from build123d import *

# Parameters (mm, degrees)
SKETCH1_W                        = 149.225
SKETCH1_H                        = 76.2
BASE_FLANGE1_DEPTH               = 3.175
EDGE_FLANGE1_STRIP_W             = 19.05
EDGE_FLANGE1_STRIP_H             = 3.175
EDGE_FLANGE1_STRIP_CUT_DEPTH     = 149.225
EDGE_FLANGE1_STRIP_2_W           = 19.05
EDGE_FLANGE1_STRIP_2_H           = 3.175
EDGE_FLANGE1_STRIP_CUT_2_DEPTH   = 149.225
EDGE_FLANGE1_DEPTH               = 149.225
EDGE_FLANGE1_BEND_DEPTH          = 149.225
SKETCH17_W                       = 25.4
SKETCH17_H                       = 9.525
CUT_EXTRUDE1_DEPTH               = 110.04244332
EDGE_FLANGE2_STRIP_W             = 19.05
EDGE_FLANGE2_STRIP_H             = 3.175
EDGE_FLANGE2_STRIP_CUT_DEPTH     = 123.825
EDGE_FLANGE2_STRIP_2_W           = 19.05
EDGE_FLANGE2_STRIP_2_H           = 3.175
EDGE_FLANGE2_STRIP_CUT_2_DEPTH   = 123.825
EDGE_FLANGE2_DEPTH               = 123.825
EDGE_FLANGE2_BEND_DEPTH          = 123.825
SKETCH18_R                       = 2.3876
CUT_EXTRUDE2_DEPTH               = 97.614069214
LPATTERN1_COUNT                  = 2
LPATTERN1_PITCH                  = 98.425
LPATTERN1_COUNT_DIR2             = 2
LPATTERN1_PITCH_DIR2             = 95.25
FILLET1_R                        = 3.175
F_10_0_1935_DIAMETER_HOLE1_D     = 4.9149
F_10_0_1935_DIAMETER_HOLE1_DEPTH = 3.175


# Sheet-metal steps are written as plain solids
with BuildPart() as part:
    # Sketch1 → Base-Flange1 (new body)
    with BuildSketch(Plane.XY):
        Rectangle(SKETCH1_W, SKETCH1_H)
    extrude(amount=-BASE_FLANGE1_DEPTH)

    # Edge-Flange1 strip (across the edge) → Edge-Flange1 strip cut (cut)
    with BuildSketch(Plane(origin=(74.6125, -38.1, -3.175), x_dir=(0, 1, 0), z_dir=(-1, 0, 0))):
        with Locations((-3.175, -1.5875)):
            Rectangle(EDGE_FLANGE1_STRIP_W, EDGE_FLANGE1_STRIP_H)
    extrude(amount=EDGE_FLANGE1_STRIP_CUT_DEPTH, mode=Mode.SUBTRACT)

    # Edge-Flange1 strip 2 (across the edge) → Edge-Flange1 strip cut 2 (cut)
    with BuildSketch(Plane(origin=(-74.6125, 38.1, -3.175), x_dir=(0, -1, 0), z_dir=(1, 0, 0))):
        with Locations((-3.175, -1.5875)):
            Rectangle(EDGE_FLANGE1_STRIP_2_W, EDGE_FLANGE1_STRIP_2_H)
    extrude(amount=EDGE_FLANGE1_STRIP_CUT_2_DEPTH, mode=Mode.SUBTRACT)

    # Edge-Flange1 section (across the edge) → Edge-Flange1 (add)
    with BuildSketch(Plane(origin=(74.6125, -38.1, -3.175), x_dir=(0, 1, 0), z_dir=(-1, 0, 0))):
        with BuildLine():
            Line((0, 3.175), (0, 19.558))
            Line((0, 19.558), (3.175, 19.558))
            Line((3.175, 19.558), (3.175, 3.175))
            ThreePointArc((3.175, 3.175), (4.10493597, 0.92993597), (6.35, 0))
            Line((6.35, 0), (6.35, -3.175))
            ThreePointArc((6.35, -3.175), (1.859871939, -1.315128061), (0, 3.175))
        make_face()
    extrude(amount=EDGE_FLANGE1_DEPTH)

    # Edge-Flange1 section 2 (across the edge) → Edge-Flange1 bend (add)
    with BuildSketch(Plane(origin=(-74.6125, 38.1, -3.175), x_dir=(0, -1, 0), z_dir=(1, 0, 0))):
        with BuildLine():
            Line((0, 3.175), (0, 19.558))
            Line((0, 19.558), (3.175, 19.558))
            Line((3.175, 19.558), (3.175, 3.175))
            ThreePointArc((3.175, 3.175), (4.10493597, 0.92993597), (6.35, 0))
            Line((6.35, 0), (6.35, -3.175))
            ThreePointArc((6.35, -3.175), (1.859871939, -1.315128061), (0, 3.175))
        make_face()
    extrude(amount=EDGE_FLANGE1_BEND_DEPTH)

    # Sketch17 → Cut-Extrude1 (cut, through all)
    with BuildSketch(Plane.XZ.offset(38.1)):
        with Locations((-61.9125, -17.9705)):
            Rectangle(SKETCH17_W, SKETCH17_H)
    extrude(amount=-CUT_EXTRUDE1_DEPTH, mode=Mode.SUBTRACT)

    # Edge-Flange2 strip (across the edge) → Edge-Flange2 strip cut (cut)
    with BuildSketch(Plane(origin=(-49.2125, -38.1, -22.733), x_dir=(0, 0, 1), z_dir=(1, 0, 0))):
        with Locations((-3.175, -1.5875)):
            Rectangle(EDGE_FLANGE2_STRIP_W, EDGE_FLANGE2_STRIP_H)
    extrude(amount=EDGE_FLANGE2_STRIP_CUT_DEPTH, mode=Mode.SUBTRACT)

    # Edge-Flange2 strip 2 (across the edge) → Edge-Flange2 strip cut 2 (cut)
    with BuildSketch(Plane(origin=(74.6125, 38.1, -22.733), x_dir=(0, 0, 1), z_dir=(-1, 0, 0))):
        with Locations((-3.175, -1.5875)):
            Rectangle(EDGE_FLANGE2_STRIP_2_W, EDGE_FLANGE2_STRIP_2_H)
    extrude(amount=EDGE_FLANGE2_STRIP_CUT_2_DEPTH, mode=Mode.SUBTRACT)

    # Edge-Flange2 section (across the edge) → Edge-Flange2 (add)
    with BuildSketch(Plane(origin=(-49.2125, -38.1, -22.733), x_dir=(0, 0, 1), z_dir=(1, 0, 0))):
        with BuildLine():
            Line((0, 3.175), (0, 18.91284))
            Line((0, 18.91284), (3.175, 18.91284))
            Line((3.175, 18.91284), (3.175, 3.175))
            ThreePointArc((3.175, 3.175), (4.10493597, 0.92993597), (6.35, 0))
            Line((6.35, 0), (6.35, -3.175))
            ThreePointArc((6.35, -3.175), (1.859871939, -1.315128061), (0, 3.175))
        make_face()
    extrude(amount=EDGE_FLANGE2_DEPTH)

    # Edge-Flange2 section 2 (across the edge) → Edge-Flange2 bend (add)
    with BuildSketch(Plane(origin=(74.6125, 38.1, -22.733), x_dir=(0, 0, 1), z_dir=(-1, 0, 0))):
        with BuildLine():
            Line((0, 3.175), (0, 18.91284))
            Line((0, 18.91284), (3.175, 18.91284))
            Line((3.175, 18.91284), (3.175, 3.175))
            ThreePointArc((3.175, 3.175), (4.10493597, 0.92993597), (6.35, 0))
            Line((6.35, 0), (6.35, -3.175))
            ThreePointArc((6.35, -3.175), (1.859871939, -1.315128061), (0, 3.175))
        make_face()
    extrude(amount=EDGE_FLANGE2_BEND_DEPTH)

    # Sketch18 → Cut-Extrude2 (cut, through all)
    with BuildSketch(Plane(origin=(0, 0, -22.733), x_dir=(-1, 0, 0), z_dir=(0, 0, -1))):
        with Locations((-61.9125, -47.48784)):
            Circle(SKETCH18_R)
    cut_extrude2 = extrude(amount=-CUT_EXTRUDE2_DEPTH, mode=Mode.SUBTRACT)

    # LPattern1: Cut-Extrude2 2 × 2
    with Locations(*[(-i * LPATTERN1_PITCH, j * LPATTERN1_PITCH_DIR2, 0) for i in range(LPATTERN1_COUNT) for j in range(LPATTERN1_COUNT_DIR2) if (i, j) != (0, 0)]):
        add(cut_extrude2, mode=Mode.SUBTRACT)

    # Fillet1
    fillet1_edges = [part.edges().sort_by_distance(p)[0] for p in [
        (-49.2125, -36.5125, -13.208),
        (-49.2125, 36.5125, -13.208),
        (-74.6125, -36.5125, -13.208),
        (-74.6125, 36.5125, -13.208),
        (-49.2125, 57.01284, -21.1455),
        (74.6125, 57.01284, -21.1455),
        (74.6125, -57.01284, -21.1455),
        (-49.2125, -57.01284, -21.1455),
    ]]
    fillet(fillet1_edges, radius=FILLET1_R)

    # #10 (0.1935) Diameter Hole1
    with Locations(Plane.XY.offset(-19.558)):
        with Locations((-36.5125, 47.76216), (61.9125, 47.76216), (61.9125, -47.48784), (-36.5125, -47.48784)):
            Hole(F_10_0_1935_DIAMETER_HOLE1_D / 2, depth=F_10_0_1935_DIAMETER_HOLE1_DEPTH)


solid = part.part
Read the model definition and answer for the solid it produces. Units are mm, in the model's axes. A direction names the side the tool comes from. Coordinates: 2 decimals unless noted, no trailing zeros. Loops run counter-clockwise (first coordinate to the right, second up) from the corner with the lowest first, then second, coordinate; pieces in that order, holes last. Notation, with made-up numbers: (33.25, -39.75) - (49.25, -39.75) arc R11 cw to (49.25, -21.75) - close; hole circle Ø5 at (11, 47.5). An arc over 180 degrees is marked (long way). Answer in a Markdown table with one row per item.
Q1. Find section D-D on x = -3.5. Write down the section's boundary in (y, z) (3 decimals), plus the area to 3 significant figures.
Here are the results:
| item | result |
|---|---|
| outline | (-57.013, -22.733) - (-41.275, -22.733) arc R6.35 ccw to (-34.925, -16.383) - (-34.925, -6.35) arc R3.175 cw to (-31.75, -3.175) - (31.75, -3.175) arc R3.175 cw to (34.925, -6.35) - (34.925, -16.383) arc R6.35 ccw to (41.275, -22.733) - (57.013, -22.733) - (57.013, -19.558) - (41.275, -19.558) arc R3.175 cw to (38.1, -16.383) - (38.1, -6.35) arc R6.35 ccw to (31.75, 0) - (-31.75, 0) arc R6.35 ccw to (-38.1, -6.35) - (-38.1, -16.383) arc R3.175 cw to (-41.275, -19.558) - (-57.013, -19.558) - close |
| area | 460 mm^2 |
Q2. Given P1, Ø4.5, axis at x = -7, y = -47.5, coming from the +Z side; P2, Ø4, axis at x = -46.5, z = -4.5, coming from the -Y side; P3, Ø2, axis at x = 53, z = -16.5, coming from the +Y side; P4, Ø8, axis at x = -36.51, y = 47.76, coming from the -Z side, each flat-ended and moving along its own axis, determine where each tip first touches the part or whether it passes through.
Here are the results:
| item | result |
|---|---|
| P1 | stops at z = -19.56 |
| P2 | stops at y = -38.1 |
| P3 | stops at y = 38.3 |
| P4 | stops at z = -22.73 |
Q3. Find section A-A on x = -58.5. Write down the section's boundary in (y, z) (3 decimals).
Here are the results:
| item | result |
|---|---|
| outline | (-38.1, -13.208) - (-34.925, -13.208) - (-34.925, -6.35) arc R3.175 cw to (-31.75, -3.175) - (31.75, -3.175) arc R3.175 cw to (34.925, -6.35) - (34.925, -13.208) - (38.1, -13.208) - (38.1, -6.35) arc R6.35 ccw to (31.75, 0) - (-31.75, 0) arc R6.35 ccw to (-38.1, -6.35) - close |
Q4. Find section C-C on y = 5.5. Write down the section's boundary in (x, z) (1 decimal).
Here are the results:
| item | result |
|---|---|
| outline | (-74.6, -3.2) - (74.6, -3.2) - (74.6, 0) - (-74.6, 0) - close |
Q5. Find section B-B on z = -8. Write down the section's boundary in (x, y) (1 decimal).
Here are the results:
| item | result |
|---|---|
| outline | (-74.6, -38.1) - (74.6, -38.1) - (74.6, -34.9) - (-74.6, -34.9) - close; (-74.6, 34.9) - (74.6, 34.9) - (74.6, 38.1) - (-74.6, 38.1) - close |
Q6. The mould has two halves that part along Y. Classify faces 6 (the flat face through (1, -38.1, -11)), 7 (the cylindrical face through (13.57, 39.05, -18.65)), 8 (the cylindrical face through (-1.04, 34.02, -4.13)): pulls with the +Y half, pulls with the -Y half, needs draft (parallel to the pull), parting line crosses it, or undercut.
Here are the results:
| item | result |
|---|---|
| face 6 | pulls with the -Y half |
| face 7 | pulls with the +Y half |
| face 8 | undercut |
Q7. For faces 1 (the cylindrical face through (13.567, 36.736, -20.823)), 2 (the cylindrical face through (-35.98, 45.363, -21.168)), 3 (the flat face through (-1, 38.1, -11)), 4 (the flat face through (-62, -37, -13.208)), 5 (the flat face through (12, -49, -19.558)), determine the directions among +Z, -Z, +X, -X, +Y, -Y from which every point of the face is accessible in a straight line to the end or side of a thin tool.
Here are the results:
| item | result |
|---|---|
| face 1 | -Z, +X, -X |
| face 2 | +Z, -Z |
| face 3 | +Z, +X, -X, +Y |
| face 4 | -Z, -X, +Y, -Y |
| face 5 | +Z, +X, -X, -Y |
Q8. Straight lines are drawn through the part: line 1 along Y through (x, z) = (-6, -15.25) (3 decimals); line 2 along Z through (x, y) = (58.5, -7.5) (3 decimals); line 3 along Z through (x, y) = (-46, 41.5). For each, find the intervals that lie inside material, in ascending order. Write a range as [from, to].
Here are the results:
| item | result |
|---|---|
| line 1 | y = [-38.1, -34.925], [34.925, 38.1] |
| line 2 | z = [-3.175, 0] |
| line 3 | z = [-22.73, -19.56] |
